```python
from build123d import *

# Parameters (mm, degrees)
BOSS_EXTRUDE1_DEPTH     = 7.9375
SKETCH3_R               = 2.032
CUT_EXTRUDE1_DEPTH      = 2.7
SKETCH4_R               = 1.000000032
CUT_EXTRUDE2_DEPTH      = 51.553064313
CUT_EXTRUDE3_DEPTH      = 52.939206859
CUT_EXTRUDE3_DEPTH_BACK = 52.939206859
CUT_EXTRUDE5_DEPTH      = 0.7
FILLET1_R               = 0.5
SKETCH6_R               = 2.032
CUT_EXTRUDE4_DEPTH      = 3.8
BOSS_EXTRUDE2_DEPTH     = 0.637


with BuildPart() as part:
    # Sketch1 → Boss-Extrude1 (new body)
    with BuildSketch(Plane(origin=(0, 0, 0), x_dir=(1, 0, 0), z_dir=(0, 1, 0))):
        Polygon((-27.620855991, -19.092445695), (-46.29298428, -16.509012872), (-42.852975587, 8.354139385), (-24.180847298, 5.770706562), align=None)
    extrude(amount=BOSS_EXTRUDE1_DEPTH)

    # Sketch3 → Cut-Extrude1 (cut)
    with BuildSketch(Plane(origin=(0.275554746, 0, -2.386974896), x_dir=(-0.9905638349724136, 0, -0.13705213914691383), z_dir=(0.13705213914691383, 0, -0.9905638349724136))):
        with Locations((40.237375061, 3.96875)):
            Circle(SKETCH3_R)
    extrude(amount=-CUT_EXTRUDE1_DEPTH, mode=Mode.SUBTRACT)

    # Sketch4 → Cut-Extrude2 (cut, through all)
    with BuildSketch(Plane(origin=(-0.040811883, 0, 0.29497369), x_dir=(-0.9905638349724136, 0, -0.13705213914691383), z_dir=(0.1370521391469138, 0, -0.9905638349724135))):
        with Locations((40.291560511, 3.96875)):
            Circle(SKETCH4_R)
    extrude(amount=-CUT_EXTRUDE2_DEPTH, mode=Mode.SUBTRACT)

    # Sketch5 → Cut-Extrude3 (cut, two sides: drawn at the far end of the back side and taken through both)
    with BuildSketch(Plane(origin=(0.329228893, 0, -2.379548664), x_dir=(-0.9905638349724137, 0, -0.1370521391469133), z_dir=(0.1370521391469133, 0, -0.9905638349724137)).offset(-CUT_EXTRUDE3_DEPTH_BACK)):
        with BuildLine():
            ThreePointArc((43.593560511, 3.96875), (42.431140549, 1.162419962), (39.624810511, 0))
            Line((39.624810511, 0), (43.593560511, 0))
            Line((43.593560511, 0), (43.593560511, 3.96875))
        make_face()
        with BuildLine():
            Line((43.593560511, 7.9375), (39.624810511, 7.9375))
            ThreePointArc((39.624810511, 7.9375), (42.431140549, 6.775080038), (43.593560511, 3.96875))
            Line((43.593560511, 3.96875), (43.593560511, 7.9375))
        make_face()
    extrude(amount=CUT_EXTRUDE3_DEPTH + CUT_EXTRUDE3_DEPTH_BACK, mode=Mode.SUBTRACT)

    # Sketch8 → Cut-Extrude5 (cut)
    with BuildSketch(Plane(origin=(-3.1107798, 0, 22.483603594), x_dir=(0.9905638349724136, 0, 0.1370521391469135), z_dir=(-0.1370521391469135, 0, 0.9905638349724137))):
        with BuildLine():
            Line((-39.624810511, 0), (-24.743560511, 0))
            Line((-24.743560511, 0), (-24.743560511, 7.9375))
            Line((-24.743560511, 7.9375), (-39.624810511, 7.9375))
            ThreePointArc((-39.624810511, 7.9375), (-43.593560511, 3.96875), (-39.624810511, 0))
        make_face()
    extrude(amount=-CUT_EXTRUDE5_DEPTH, mode=Mode.SUBTRACT)

    # Fillet1
    fillet1_edges = [part.edges().sort_by_distance(p)[0] for p in [
        (-42.852975587, 3.96875, -8.354139385),
        (-31.551261333, 0, -6.790460135),
        (-46.197047782, 3.96875, 15.815618188),
        (-34.895333528, 7.9375, 17.379297438),
        (-34.895333528, 0, 17.379297438),
        (-31.551261333, 7.9375, -6.790460135),
    ]]
    fillet(fillet1_edges, radius=FILLET1_R)

    # Sketch6 → Cut-Extrude4 (cut)
    # profile 1 of 4: a face of its own
    with BuildSketch(Plane(origin=(0.329228893, 0, -2.379548664), x_dir=(-0.9905638349724137, 0, -0.1370521391469133), z_dir=(0.1370521391469133, 0, -0.9905638349724137))):
        with BuildLine():
            Line((41.099755957, 7.039164487), (39.857545305, 7.366139557))
            Line((39.857545305, 7.366139557), (26.117003817, 5.610790678))
            ThreePointArc((26.117003817, 5.610790678), (25.770140702, 3.96875), (26.117003817, 2.326709322))
            Line((26.117003817, 2.326709322), (39.857545305, 0.571360443))
            Line((39.857545305, 0.571360443), (41.099755957, 0.898335513))
            ThreePointArc((41.099755957, 0.898335513), (40.498298253, 0.800487936), (39.889225247, 0.819345082))
            Line((39.889225247, 0.819345082), (26.291560511, 2.556441511))
            Line((26.291560511, 2.556441511), (26.291560511, 3.67018175))
            ThreePointArc((26.291560511, 3.67018175), (27.210560511, 3.96875), (26.291560511, 4.26731825))
            Line((26.291560511, 4.26731825), (26.291560511, 5.381058489))
            Line((26.291560511, 5.381058489), (39.889225247, 7.118154918))
            ThreePointArc((39.889225247, 7.118154918), (40.498298253, 7.137012064), (41.099755957, 7.039164487))
        make_face()
    # profile 2 of 4: a face of its own
    with BuildSketch(Plane(origin=(0.329228893, 0, -2.379548664), x_dir=(-0.9905638349724137, 0, -0.1370521391469133), z_dir=(0.1370521391469133, 0, -0.9905638349724137))):
        with BuildLine():
            ThreePointArc((39.889225247, 0.819345082), (37.116560511, 3.96875), (39.889225247, 7.118154918))
            Line((39.889225247, 7.118154918), (26.291560511, 5.381058489))
            Line((26.291560511, 5.381058489), (26.291560511, 4.26731825))
            ThreePointArc((26.291560511, 4.26731825), (27.210560511, 3.96875), (26.291560511, 3.67018175))
            Line((26.291560511, 3.67018175), (26.291560511, 2.556441511))
            Line((26.291560511, 2.556441511), (39.889225247, 0.819345082))
        make_face()
    # profile 3 of 4: a face of its own
    with BuildSketch(Plane(origin=(0.329228893, 0, -2.379548664), x_dir=(-0.9905638349724137, 0, -0.1370521391469133), z_dir=(0.1370521391469133, 0, -0.9905638349724137))):
        with BuildLine():
            ThreePointArc((41.421703743, 6.935802624), (41.262106814, 6.991772473), (41.099755957, 7.039164487))
            ThreePointArc((41.099755957, 7.039164487), (40.498298253, 7.137012064), (39.889225247, 7.118154918))
            ThreePointArc((39.889225247, 7.118154918), (37.116560511, 3.96875), (39.889225247, 0.819345082))
            ThreePointArc((39.889225247, 0.819345082), (40.498298253, 0.800487936), (41.099755957, 0.898335513))
            ThreePointArc((41.099755957, 0.898335513), (41.262106814, 0.945727527), (41.421703743, 1.001697376))
            ThreePointArc((41.421703743, 1.001697376), (43.093560511, 3.96875), (41.421703743, 6.935802624))
        make_face()
        with Locations((40.291560511, 3.96875)):
            Circle(SKETCH6_R, mode=Mode.SUBTRACT)
    # profile 4 of 4: a face of its own
    with BuildSketch(Plane(origin=(0.329228893, 0, -2.379548664), x_dir=(-0.9905638349724137, 0, -0.1370521391469133), z_dir=(0.1370521391469133, 0, -0.9905638349724137))):
        with Locations((40.291560511, 3.96875)):
            Circle(SKETCH6_R)
    extrude(amount=-CUT_EXTRUDE4_DEPTH, mode=Mode.SUBTRACT)

    # Sketch7 → Boss-Extrude2 (add)
    with BuildSketch(Plane(origin=(-24.510076191, 0, -3.391157898), x_dir=(0.13705213914691317, 0, -0.9905638349724137), z_dir=(0.9905638349724137, 0, 0.13705213914691317))):
        with BuildLine():
            Line((-21.497783626, 0), (1.902216374, 0))
            ThreePointArc((1.902216374, 0), (2.255769765, 0.146446609), (2.402216374, 0.5))
            Line((2.402216374, 0.5), (2.402216374, 7.4375))
            ThreePointArc((2.402216374, 7.4375), (2.255769765, 7.791053391), (1.902216374, 7.9375))
            Line((1.902216374, 7.9375), (-21.497783626, 7.9375))
            ThreePointArc((-21.497783626, 7.9375), (-21.851337016, 7.791053391), (-21.997783626, 7.4375))
            Line((-21.997783626, 7.4375), (-21.997783626, 0.5))
            ThreePointArc((-21.997783626, 0.5), (-21.851337016, 0.146446609), (-21.497783626, 0))
        make_face()
    extrude(amount=BOSS_EXTRUDE2_DEPTH)


solid = part.part
```
The listing builds one solid part. Answer for the finished solid, in the listing's coordinates (mm). A direction names the side the tool comes from. Give positions to 0.01 mm unless a question says otherwise; leave off trailing zeros.
Item 1: Find the intervals of material crossed by probe 1 along X at (y, z) = (5, -5.5); probe 2 along Z at (x, y) = (-30.25, 1.25); probe 3 along X at (y, z) = (5.5, 14), in increasing order.
From the geometry:
probe 1: x = -43.11 to -42.58, -25.39 to -23.58
probe 2: z = -6.61 to 18.02
probe 3: x = -45.64 to -26.27
Item 2: For a pull along Y with two mould halves and no side action, classify faces 4 (the face through (-40.798, 0.945, -6.179)), 5 (the face through (-34.667, 7.795, 17.259)), 6 (the face through (-25.245, 4.024, 6.571)) as pulls with the +Y half, pulls with the -Y half, needs draft (parallel to the pull), parting line crosses it, or undercut.
From the geometry:
face 4: undercut
face 5: pulls with the +Y half
face 6: needs draft
Item 3: Which of the six approach directions +Z, -Z, +X, -X, +Y, -Y give full straight-line access (tool end or side, diameter ignored) to faces 1 (the face through (-25.455, 3.992, -4.056)), 2 (the face through (-36.43, 4.017, 17.167)), 3 (the face through (-42.614, 3.919, -6.43))?
From the geometry:
face 1: -Z
face 2: +Z, -X, +Y, -Y
face 3: none
Item 4: The part is cut by section A-A, the plane z = -3.5. Count the separate pieces of the cut face and the enclosed holes in it, and give its area (3 significant figures).
From the geometry:
separate pieces: 1
enclosed holes: 2
area: 102 mm2
Item 5: Given pin 1 Ø4 at (x, y) = (-39, 7) entering from -Z; pin 2 Ø4 at (y, z) = (3.5, 7.5) entering from +X; pin 3 Ø3 at (y, z) = (5, 4) entering from -X, each flat-ended and moving along its own axis, determine where each tip first touches the part or whether it passes through.
From the geometry:
pin 1: stops at z = -8.1
pin 2: stops at x = -25.1
pin 3: stops at x = -44.73
